Read the model definition and answer for the solid it produces. Units are mm, in the model's axes. Face numbers are marked on the shaded views. A direction names the side the tool comes from. Round coordinates to 2 decimals unless told otherwise and drop trailing zeros. Write each loop counter-clockwise with the first axis right and the second up, starting at its lowest first coordinate (ties: lowest second). Pieces come first, ordered by that corner, then holes. Notation, with made-up numbers: (64, -10.5) -> (70, -10.5) arc R15 ccw to (70, -5.5) -> close; hole circle Ø11 at (81.5, 9.25). An arc over 180 degrees is marked (long way). Return JSON: item names as keys, results as strings. Group by question number.
(1) For the marked faces 4, 5 and 6, determine the directions among +Z, -Z, +X, -X, +Y, -Y from which every point of the face is accessible in a straight line to the end or side of a thin tool.
(2) A cutting plane is placed at B-B on z = 36.5. Give the vertices of the cut face in (x, y).
(3) A cutting plane is placed at D-D on y = -914. Give the vertices of the cut face in (x, z), then the cut area to 3 significant figures.
(4) Given pin 1 (4 mm diameter, centred on x = 203, z = -91.5, fed in from +Y) (3 decimals), flat-ended and moving along its own axis, determine where the tip first touches the part or whether it passes through.
(5) A cutting plane is placed at C-C on z = -237. Give the vertices of the cut face in (x, y), then the cut area to 3 significant figures.
(6) Straight lines are drawn through the part: line 1 (Z direction, x = -459.5, y = -197); line 2 (Y direction, x = 0, z = 772); line 3 (Z direction, x = -43.5, y = -619.5). For each, find the intervals that lie inside material, in ascending order.
(7) The mould has two halves that part along Y. Classify the marked faces 1, 2 and 3: released by +Y, released by -Y, zero draft, split by the parting line, or undercut.
(8) A cutting plane is placed at A-A on y = -1165.5. Give the vertices of the cut face in (x, z).
```python
from build123d import *

# Parameters (mm, degrees)
F0_W     = 1701.8
F0_H     = 1701.8
F1_DEPTH = 1422.4
F3_DEPTH = 38.1
F4_W     = 736.6
F4_H     = 83.82
F5_DEPTH = 1950.72
F7_DEPTH = 2123.44
F9_DEPTH = 383.54


with BuildPart() as f1:
    # F0 (on Front) → F1 (new body)
    with BuildSketch(Plane.XZ):
        Rectangle(F0_W, F0_H)
    extrude(amount=F1_DEPTH)

    # F2 (on face) → F3 (cut)
    with BuildSketch(Plane.XZ.offset(1422.4)):
        Polygon((-850.9, 678.4790824755), (-172.4209175245, 0), (0, 172.4209175245), (-678.4790824755, 850.9), (-850.9, 850.9), align=None)
        Polygon((-172.4209175245, 0), (-850.9, -678.4790824755), (-850.9, -850.9), (-678.4790824755, -850.9), (0, -172.4209175245), align=None)
        Polygon((0, 172.4209175245), (-172.4209175245, 0), (0, -172.4209175245), (172.4209175245, 0), align=None)
        Polygon((678.4790824755, 850.9), (0, 172.4209175245), (172.4209175245, 0), (850.9, 678.4790824755), (850.9, 850.9), align=None)
        Polygon((172.4209175245, 0), (0, -172.4209175245), (678.4790824755, -850.9), (850.9, -850.9), (850.9, -678.4790824755), align=None)
    extrude(amount=-F3_DEPTH, mode=Mode.SUBTRACT)

    # F4 (on face) → F5 (cut)
    with BuildSketch(Plane.YZ.offset(850.9)):
        with Locations((-368.3, 491.49)):
            Rectangle(F4_W, F4_H)
    extrude(amount=-F5_DEPTH, mode=Mode.SUBTRACT)

    # F6 (on face) → F7 (cut)
    with BuildSketch(Plane.YZ.offset(850.9)):
        with BuildLine():
            ThreePointArc((-322.7768453567, -482.6), (-274.564901456, -366.2060711665), (-258.1207052231, -241.3))
            ThreePointArc((-258.1207052231, -241.3), (-274.564901456, -116.3939288335), (-322.7768453567, 0))
            Line((-322.7768453567, 0), (-740.7207052231, 0))
            Line((-740.7207052231, 0), (-740.7207052231, -241.3))
            Line((-740.7207052231, -241.3), (-740.7207052231, -482.6))
            Line((-740.7207052231, -482.6), (-322.7768453567, -482.6))
        make_face()
        with BuildLine():
            ThreePointArc((-322.7768453567, 0), (-274.564901456, -116.3939288335), (-258.1207052231, -241.3))
            ThreePointArc((-258.1207052231, -241.3), (-274.564901456, -366.2060711665), (-322.7768453567, -482.6))
            Line((-322.7768453567, -482.6), (76.7071917653, -482.6))
            Line((76.7071917653, -482.6), (76.7071917653, 0))
            Line((76.7071917653, 0), (-322.7768453567, 0))
        make_face()
        with BuildLine():
            Line((-740.7207052231, 0), (-322.7768453567, 0))
            ThreePointArc((-322.7768453567, 0), (-1223.3207052231, -241.3), (-322.7768453567, -482.6))
            Line((-322.7768453567, -482.6), (-740.7207052231, -482.6))
            Line((-740.7207052231, -482.6), (-740.7207052231, -241.3))
            Line((-740.7207052231, -241.3), (-740.7207052231, 0))
        make_face()
    extrude(amount=-F7_DEPTH, mode=Mode.SUBTRACT)

    # F8 (on face) → F9 (cut)
    with BuildSketch(Plane.XY.offset(850.9)):
        with BuildLine():
            ThreePointArc((0, -130.81), (-56.5756135627, -267.3956135627), (80.01, -210.82))
            ThreePointArc((80.01, -210.82), (56.5756135627, -154.2443864373), (0, -130.81))
        make_face()
    extrude(amount=-F9_DEPTH, mode=Mode.SUBTRACT)


solid = f1.part
```
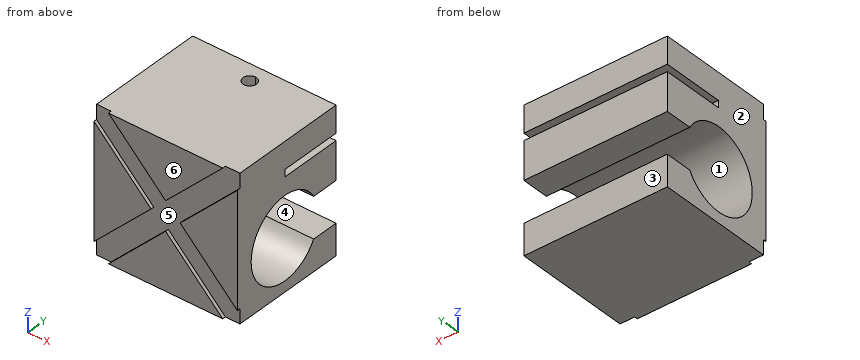
Checks:
{
 "1": {"face 4": "+X, -X, +Y", "face 5": "-Y", "face 6": "+Z, -Z, +X, -X, -Y"},
 "2": {"outline": "(-850.9, -1422.4) -> (-208.92, -1422.4) -> (-208.92, -1384.3) -> (208.92, -1384.3) -> (208.92, -1422.4) -> (850.9, -1422.4) -> (850.9, -1135.35) -> (-850.9, -1135.35) -> close; (-850.9, -346.09) -> (850.9, -346.09) -> (850.9, 0) -> (-850.9, 0) -> close"},
 "3": {"outline": "(-850.9, -850.9) -> (850.9, -850.9) -> (850.9, -691.72) -> (-850.9, -691.72) -> close; (-850.9, 209.12) -> (850.9, 209.12) -> (850.9, 850.9) -> (-850.9, 850.9) -> close", "area": "1,360,000 mm^2"},
 "4": {"pin 1": "stops at y = -1198.825"},
 "5": {"outline": "(-850.9, -1422.4) -> (-409.42, -1422.4) -> (-409.42, -1384.3) -> (-64.58, -1384.3) -> (-64.58, -1422.4) -> (64.58, -1422.4) -> (64.58, -1384.3) -> (409.42, -1384.3) -> (409.42, -1422.4) -> (850.9, -1422.4) -> (850.9, -1223.3) -> (-850.9, -1223.3) -> close", "area": "313,000 mm^2"},
 "6": {"line 1": "z = -850.9 to -482.6, 0 to 449.58, 533.4 to 850.9", "line 2": "y = -1422.4 to -290.83, -130.81 to 0", "line 3": "z = -850.9 to -708.43, 225.83 to 449.58, 533.4 to 850.9"},
 "7": {"face 1": "undercut", "face 2": "zero draft", "face 3": "released by +Y"},
 "8": {"outline": "(-850.9, -850.9) -> (850.9, -850.9) -> (850.9, -470.35) -> (-850.9, -470.35) -> close; (-850.9, -12.25) -> (850.9, -12.25) -> (850.9, 850.9) -> (-850.9, 850.9) -> close"}
}
